```python
from build123d import *

# Parameters (mm, degrees)
F1_DEPTH = 25
F3_DEPTH = 71.0393057594
F4_DEPTH = 25


with BuildPart() as f1:
    # F0 (on Right) → F1 (new body)
    with BuildSketch(Plane.YZ):
        Polygon((0, 10.2), (0, 0), (10, 0), (60, 0), (60, 10.2), align=None)
        Polygon((10, 0), (0, 0), (0, -10.2), (10, -10.2), (10, -5.4790303111), align=None)
        with BuildLine():
            Line((12.9808050988, -2.4790917191), (10, 0))
            Line((10, 0), (10, -5.4790303111))
            ThreePointArc((10, -5.4790303111), (10.8719040549, -3.3645072802), (12.9808050988, -2.4790917191))
        make_face()
        Polygon((0, 30.3931459785), (0, 10.2), (60, 10.2), (71.0383057594, 10.2), (71.0383057594, 30.3931459785), align=None)
        with BuildLine():
            ThreePointArc((13.4366949561, -8.4470763881), (11.0391436652, -7.7495021639), (10, -5.4790303111))
            Line((10, -5.4790303111), (10, -10.2))
            Line((10, -10.2), (13.4366949561, -8.4470763881))
        make_face()
    extrude(amount=F1_DEPTH)

    # F2 (on face) → F3 (cut, through all)
    with BuildSketch(Plane.XZ):
        with BuildLine():
            ThreePointArc((10.1552814897, 10), (6.1552813277, 12.0000002161), (2.1552811656, 10))
            Line((2.1552811656, 10), (10.1552814897, 10))
        make_face()
        with BuildLine():
            ThreePointArc((2.1552811656, 10), (1.1888790402, 7.5786610142), (1.572705727, 5))
            Line((1.572705727, 5), (10.7378569283, 5))
            ThreePointArc((10.7378569283, 5), (11.0498128682, 5.9784518822), (11.1552813277, 7.0000002161))
            ThreePointArc((11.1552813277, 7.0000002161), (10.8986978606, 8.581138918), (10.1552814897, 10))
            Line((10.1552814897, 10), (2.1552811656, 10))
        make_face()
        with BuildLine():
            Line((10.7378569283, 5), (1.572705727, 5))
            ThreePointArc((1.572705727, 5), (6.1552813277, 2.0000002161), (10.7378569283, 5))
        make_face()
        with BuildLine():
            Line((14.9572591335, 10), (22.9572591335, 10))
            ThreePointArc((22.9572591335, 10), (18.9572591335, 12), (14.9572591335, 10))
        make_face()
        with BuildLine():
            Line((14.3746834385, 5), (23.5398348284, 5))
            ThreePointArc((23.5398348284, 5), (23.8517906981, 5.9784517816), (23.9572591335, 7))
            ThreePointArc((23.9572591335, 7), (23.7006756237, 8.5811388301), (22.9572591335, 10))
            Line((22.9572591335, 10), (14.9572591335, 10))
            ThreePointArc((14.9572591335, 10), (13.9908568753, 7.5786610494), (14.3746834385, 5))
        make_face()
        with BuildLine():
            ThreePointArc((14.3746834385, 5), (18.9572591335, 2), (23.5398348284, 5))
            Line((23.5398348284, 5), (14.3746834385, 5))
        make_face()
    extrude(amount=-F3_DEPTH, mode=Mode.SUBTRACT)

    # F4 (add): a face of the model
    f4_faces = [f1.faces().sort_by_distance(p)[0] for p in [
        (12.4896952291, 0, 10.6636485804),
    ]]
    extrude(f4_faces, amount=F4_DEPTH)


solid = f1.part
```
Source: CAD feature listing. Evaluate the final solid. Frame: model axes, mm. A direction names the side the tool comes from. Round coordinates to 2 decimals unless told otherwise and drop trailing zeros. Write each loop counter-clockwise with the first axis right and the second up, starting at its lowest first coordinate (ties: lowest second). Pieces come first, ordered by that corner, then holes. Notation, with made-up numbers: M 12,66 L 66,66 A15 ccw 66,77 Z; hole C 68,68.25 d8. An arc over 180 degrees is marked long. Answer as a JSON object with one key per item and string values. Group by question number.
(1) Section query B-B on z = 4. Output: boundary loops of the cut face in (x, y), then the cut area to 3 significant figures.
(2) Section query D-D on x = 12.5. Output: boundary loops of the cut face in (y, z), then the cut area to 3 significant figures.
(3) Reachability of faces 1 (the flat face through (12, -7, -10.2)), 2 (the flat face through (1, 65, 10.2)) from +Z, -Z, +X, -X, +Y, -Y: full face, straight path, thin tool, end or side. Return the list, or none.
(4) First-contact query: pin 1 (1 mm diameter, centred on x = 18.5, y = 15.5, fed in from -Z); pin 2 (1.5 mm diameter, centred on x = 11.5, y = 65.5, fed in from -Z). Flat tips, straight axial feed; report the tip coordinate or a pass-through.
(5) Ray query, line 1 (X direction, y = 18.5, z = 4); line 2 (X direction, y = 13.5, z = 6.5); line 3 (Z direction, x = 22, y = -11). Return the intervals inside material, ascending. Write a range as [from, to].
(6) Section query C-C on x = 19.5. Output: boundary loops of the cut face in (y, z), then the cut area to 3 significant figures.
(7) Section query A-A on y = 29.5. Output: boundary loops of the cut face in (x, z).
Computed values:
{
 "1": {"outline": "M 0,-25 L 2.16,-25 L 2.16,60 L 0,60 Z; M 10.16,-25 L 14.96,-25 L 14.96,60 L 10.16,60 Z; M 22.96,-25 L 25,-25 L 25,60 L 22.96,60 Z", "area": "765 mm^2"},
 "2": {"outline": "M -25,-10.2 L 10,-10.2 L 13.44,-8.45 A3 cw long 12.98,-2.48 L 10,0 L 60,0 L 60,10.2 L 71.04,10.2 L 71.04,30.39 L -25,30.39 Z", "area": "3,170 mm^2"},
 "3": {"face 1": "-Z, +X, -X, +Y, -Y", "face 2": "-Z, +X, -X, +Y"},
 "4": {"pin 1": "z = 0", "pin 2": "z = 10.2"},
 "5": {"line 1": "[0, 2.16], [10.16, 14.96], [22.96, 25]", "line 2": "[0, 1.18], [11.13, 13.98], [23.93, 25]", "line 3": "[-10.2, 3.03], [10.97, 30.39]"},
 "6": {"outline": "M -25,-10.2 L 10,-10.2 L 13.44,-8.45 A3 cw long 12.98,-2.48 L 10,0 L 60,0 L 60,2.03 L -25,2.03 Z; M -25,11.97 L 71.04,11.97 L 71.04,30.39 L -25,30.39 Z", "area": "2,310 mm^2"},
 "7": {"outline": "M 0,0 L 25,0 L 25,30.39 L 0,30.39 Z; hole C 6.16,7 d10; hole C 18.96,7 d10"}
}
